```python
from build123d import *

# Parameters (mm, degrees)
F0_W     = 10
F0_H     = 10
F1_DEPTH = 20
F2_DEPTH = 10


with BuildPart() as f1:
    # F0 (on Top) → F1 (new body)
    with BuildSketch(Plane.XY):
        with Locations((-15, 5)):
            Rectangle(F0_W, F0_H)
    extrude(amount=F1_DEPTH)

    # F0 (on Top) → F2 (join)
    with BuildSketch(Plane.XY):
        with Locations((-5, 15)):
            Rectangle(F0_W, F0_H)
        with Locations((-5, 5)):
            Rectangle(F0_W, F0_H)
    extrude(amount=F2_DEPTH)


solid = f1.part
```
The listing builds one solid part. Answer for the finished solid, in the listing's coordinates (mm). A direction names the side the tool comes from. Give positions to 0.01 mm unless a question says otherwise; leave off trailing zeros. Order: outer loops, then holes, each group sorted by start corner. A loop starts at its lowest first (then second) coordinate and runs counter-clockwise, first axis right, second up. Notation, with made-up numbers: (-11.75, 80) -> (18.25, 80) arc R14 ccw to (18.25, 93) -> close; hole circle Ø7 at (34.25, 38). An arc over 180 degrees is marked (long way). Answer as a JSON object with one key per item and string values. Group by question number.
Item 1: The part is cut by section A-A on z = 2.25. Write down the section's boundary in (x, y), and give its area (3 significant figures).
Item 2: The part is cut by section D-D on y = 13.5. Write down the section's boundary in (x, z), and give its area (3 significant figures).
Item 3: A tool of negligible diameter and unlimited length cuts with its end or side. For faces 1 (the flat face through (-15, 10, 10)), 2 (the flat face through (-12, 0, 8)), 3 (the flat face through (-5, 10, 10)), from which of +Z, -Z, +X, -X, +Y, -Y can it reach the whole face along a straight path? Write none if from no direction.
Item 4: Flat-ended cylindrical pins translate along their axes: pin 1 (10 mm diameter, centred on y = 11.5, z = 11, fed in from +X); pin 2 (5 mm diameter, centred on x = -15, z = 14.5, fed in from +Y); pin 3 (3 mm diameter, centred on y = 14.5, z = 4, fed in from -X); pin 4 (6 mm diameter, centred on x = -5.5, y = 17, fed in from +Z). Find the tip coordinate at first contact, or state that the pin passes through.
Item 5: The part is cut by section B-B on y = 2. Write down the section's boundary in (x, z).
Item 6: The part is cut by section C-C on x = -13.5. Write down the section's boundary in (y, z), and give its area (3 significant figures).
Item 7: Consider L1, parallel to Y at x = -16.25, z = 1; L2, parallel to X at y = 2.5, z = 18; L3, parallel to X at y = 18.25, z = 5. Determine where each line is inside the solid, lowest interval first. Write a range as from..to.
Result set:
{
 "1": {"outline": "(-20, 0) -> (0, 0) -> (0, 20) -> (-10, 20) -> (-10, 10) -> (-20, 10) -> close", "area": "300 mm²"},
 "2": {"outline": "(-10, 0) -> (0, 0) -> (0, 10) -> (-10, 10) -> close", "area": "100 mm²"},
 "3": {"face 1": "+Z, -Z, -X, +Y", "face 2": "+Z, -Z, +X, -X, -Y", "face 3": "+Z, +X, +Y, -Y"},
 "4": {"pin 1": "x = 0", "pin 2": "y = 10", "pin 3": "x = -10", "pin 4": "z = 10"},
 "5": {"outline": "(-20, 0) -> (0, 0) -> (0, 10) -> (-10, 10) -> (-10, 20) -> (-20, 20) -> close"},
 "6": {"outline": "(0, 0) -> (10, 0) -> (10, 20) -> (0, 20) -> close", "area": "200 mm²"},
 "7": {"L1": "0..10", "L2": "-20..-10", "L3": "-10..0"}
}
